Source: CAD feature listing. Evaluate the final solid. Frame: model axes, mm. Face numbers are marked on the shaded views. A direction names the side the tool comes from. Coordinates: 2 decimals unless noted, no trailing zeros. Order: outer loops, then holes, each group sorted by start corner. A loop starts at its lowest first (then second) coordinate and runs counter-clockwise, first axis right, second up.
Item 1: Contact query for flat-ended pins moving along their axis: P1, Ø15.5, axis at x = -13.5, z = 5, coming from the +Y side; P2, Ø6, axis at x = -32, z = 5, coming from the -Y side; P3, Ø15.5, axis at x = -18, z = 41.5, coming from the +Y side; P4, Ø2, axis at x = 1, y = 8, coming from the -Z side. Output: stop coordinate, or through.
Item 2: Section A-A on x = -32. Return the cut outline in (y, z).
Item 3: Section D-D on x = 19.5. Return the cut outline in (y, z).
Item 4: Ray query, line 1 (Z direction, x = -32, y = 2.3); line 2 (Z direction, x = 12.5, y = 9.5); line 3 (Y direction, x = -35.5, z = 13.5). Return the intervals inside material, ascending.
Item 5: Reachability of the marked faces 1, 2, 3, 4 and 5 from +Z, -Z, +X, -X, +Y, -Y: full face, straight path, thin tool, end or side. Return the list, or none.
Item 6: Section C-C on y = 2. Return the cut outline in (x, z).
Item 7: Section B-B on z = 25. Return the cut outline in (x, y), then the cut area to 3 significant figures.
Autodesk Inventor part; units mm, degrees
ref_plane "Work Plane1" through (-0.529, 3, 0) normal (0.9848078, 0.1736482, 0) x (0, 0, -1)
ref_plane "YZ Plane" through (0, 0, 0) normal (1, 0, 0) x (0, 1, 0)
ref_plane "XZ Plane" through (0, 0, 0) normal (0, 1, 0) x (-1, 0, 0)
sketch "Sketch1" plane through (0, 0, 0) normal (0, 0, 1) x (1, 0, 0)
  line L0 (0, 0) -> (-40, 0)
  line L1 (-40, 0) -> (-40, 3)
  line L2 (-40, 3) -> (0, 3)
  line L3 (0, 3) -> (0, 0)
  line L4 (0, 0) -> (-1.0261, 2.8191)
  line L5 (-1.0261, 2.8191) -> (36.5616, 16.4999)
  line L6 (36.5616, 16.4999) -> (37.5877, 13.6808)
  line L7 (37.5877, 13.6808) -> (0, 0)
  point P0 (-0.529, 3)
  dimension "d0" = 160
  dimension "d1" = 3
  dimension "d2" = 3
  dimension "d3" = 40
  dimension "d4" = 40
extrude "Extrusion1" add sketch "Sketch1" along normal blind 50
sketch "Sketch2" plane through (-40, 3, 0) normal (0, 1, 0) x (1, 0, 0)
  line L0 (0, 0) -> (40, 0)
  line L1 (0, -50) -> (40, -50)
  circle A0 centre (8, -45) radius 2.25
  circle A1 centre (8, -25) radius 2.25
  circle A2 centre (8, -5) radius 2.25
  line L2 (8, 0) -> (8, -50)
  line L3 (0, 0) -> (0, -50)
  point P0 (8, -25)
  dimension "d7" = 4.5
  dimension "d8" = 4.5
  dimension "d9" = 4.5
  dimension "d10" = 20
  dimension "d12" = 8
  dimension "d13" = 20
extrude "Extrusion2" cut sketch "Sketch2" against normal blind 50 contours L2 A2 | A2 L2 | L2 A0 | A0 L2 | L2 A1 | A1 L2
ref_plane "Work Plane1" through (-0.529, 3, 0) normal (0.9848078, 0.1736482, 0) x (0, 0, -1)
mirror "Mirror1" about plane through (-0.529, 3, 0) normal (0.9848078, 0.1736482, 0) of "Extrusion2"
fillet "Fillet1" radius 5 4 edges at (37.0747, 15.0903, 0) (37.0747, 15.0903, 50) (-40, 1.5, 50) (-40, 1.5, 0)
sketch "Sketch3" plane through (-0.529, 3, 0) normal (0.9848078, 0.1736482, 0) x (0, 0, -1)
  line L0 (-5, 6.8541) -> (-45, 6.8541)
  ellipse E0 centre (-45, 5.4649) end of major axis (-47.25, 5.4649) minor radius 0.3907
  ellipse E1 centre (-25, 5.4649) end of major axis (-27.25, 5.4649) minor radius 0.3907
  ellipse E2 centre (-5, 5.4649) end of major axis (-7.25, 5.4649) minor radius 0.3907
  line L1 (-25, 5.4649) -> (-25, 19.1248)
  line L2 (-45, 5.4649) -> (-25, 5.4649)
  line L3 (-36, -8.762) -> (-34, -8.762)
  line L4 (-34, -8.762) -> (-34, 19.6918)
  line L5 (-34, 19.6918) -> (-36, 19.6918)
  line L6 (-36, 19.6918) -> (-36, -8.762)
  line L7 (-36, -8.762) -> (-34, 19.6918) construction
  line L8 (-34, -8.762) -> (-36, 19.6918) construction
  ellipse E3 centre (-5, 5.9858) end of major axis (0, 5.9858) minor radius 0.8682 (0, 5.9858) -> (-5, 6.8541) ccw
  line L9 (-5, 6.8541) -> (-45, 6.8541)
  ellipse E4 centre (-45, 5.9858) end of major axis (-40, 5.9858) minor radius 0.8682 (-45, 6.8541) -> (-50, 5.9858) ccw
  line L10 (-50, 0) -> (-50, 5.9858)
  line L11 (0, 0) -> (-50, 0)
  line L12 (0, 0) -> (0, 5.9858)
  ellipse E5 centre (-45, 5.4649) end of major axis (-47.25, 5.4649) minor radius 0.3907
  ellipse E6 centre (-25, 5.4649) end of major axis (-27.25, 5.4649) minor radius 0.3907
  ellipse E7 centre (-5, 5.4649) end of major axis (-7.25, 5.4649) minor radius 0.3907
  line L13 (-14, -8.762) -> (-16, -8.762)
  line L14 (-16, -8.762) -> (-16, 19.6918)
  line L15 (-16, 19.6918) -> (-14, 19.6918)
  line L16 (-14, 19.6918) -> (-14, -8.762)
  line L17 (-14, -8.762) -> (-16, 19.6918) construction
  line L18 (-16, -8.762) -> (-14, 19.6918) construction
  point P0 (0, -3.0463)
  point P1 (-35, 5.4649)
  point P2 (-15, 5.4649)
  point P3 (-14, 0)
  point P4 (-14, 6.8541)
  point P5 (-16, 6.8541)
  point P6 (-16, 0)
  point P7 (-36, 0)
  point P8 (-34, 0)
  point P9 (-34, 6.8541)
  point P10 (-36, 6.8541)
  dimension "d17" = 2
extrude "Extrusion3" add sketch "Sketch3" against normal up to next contours L16 L11 L14 L0 | L4 L2 L6 L0 | L11 L6 L2 L4
mirror "Mirror2" about plane through (-0.529, 3, 0) normal (0.9848078, 0.1736482, 0) of "Extrusion3"
sketch "Sketch4" plane through (-0.529, 3, 34) normal (-0.3420201, 0.9396926, 0) x (0.9396926, 0.3420201, 0)
  circle A0 centre (13.7993, 29) radius 2.25
  circle A1 centre (13.7993, 9) radius 2.25
  circle A2 centre (13.7993, -11) radius 2.25
  point P0 (-0.529, 34)
extrude "Extrusion4" cut sketch "Sketch4" against normal blind 10
properties part number "Angle_3DPrint"
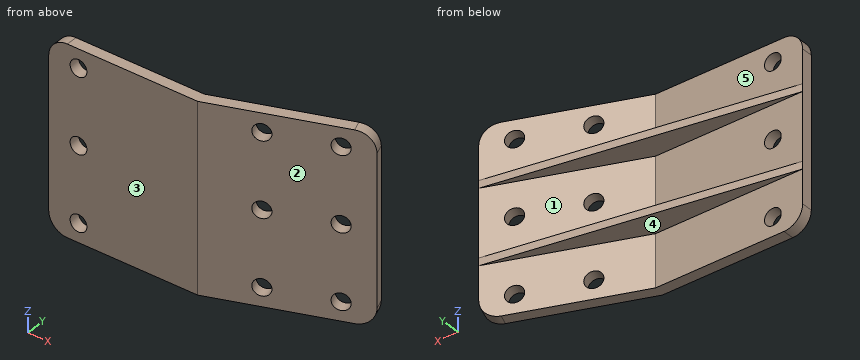
Answer list:
1. P1: stops at y = 3
1. P2: stops at y = 0
1. P3: stops at y = 7.84
1. P4: stops at z = 14
2. outline: (0, 0) - (3, 0) - (3, 2.75) - (0, 2.75) - close; (0, 7.25) - (3, 7.25) - (3, 14) - (4.41, 14) - (4.41, 16) - (3, 16) - (3, 22.75) - (0, 22.75) - close; (0, 27.25) - (3, 27.25) - (3, 34) - (4.41, 34) - (4.41, 36) - (3, 36) - (3, 42.75) - (0, 42.75) - close; (0, 47.25) - (3, 47.25) - (3, 50) - (0, 50) - close
3. outline: (7.1, 0) - (10.29, 0) - (10.29, 14) - (13.49, 14) - (13.49, 16) - (10.29, 16) - (10.29, 34) - (13.49, 34) - (13.49, 36) - (10.29, 36) - (10.29, 50) - (7.1, 50) - close
4. line 1: z = 0 to 2.75, 7.25 to 22.75, 27.25 to 42.75, 47.25 to 50
4. line 2: z = 14 to 16, 34 to 36
4. line 3: y = 0 to 3
5. face 1: -X, +Y
5. face 2: +Z, -Z, +X, -Y
5. face 3: +Z, -Z, +X, -X, -Y
5. face 4: -Z, -X, +Y
5. face 5: +Z, -X, +Y
6. outline: (-40, 5) arc R5 ccw to (-35, 0) - (5.49, 0) - (5.49, 50) - (-35, 50) arc R5 ccw to (-40, 45) - close; hole circle Ø4.5 at (-32, 5); hole circle Ø4.5 at (-32, 25); hole circle Ø4.5 at (-32, 45)
7. outline: (-40, 0) - (-34.25, 0) - (-34.25, 3) - (-40, 3) - close; (-29.75, 0) - (0, 0) - (11.35, 4.13) - (10.32, 6.95) - (-0.53, 3) - (-29.75, 3) - close; (14.55, 8.49) - (15.58, 5.67) - (27.96, 10.18) - (26.93, 12.99) - close; (31.16, 14.53) - (32.18, 11.71) - (37.59, 13.68) - (36.56, 16.5) - close
7. area: 198 mm2
